Can you work these out from the model? Positions are in its coordinate system, mm. Face numbers are marked on the shaded views. A direction names the side the tool comes from. Coordinates: 2 decimals unless noted, no trailing zeros. Loops run counter-clockwise (first coordinate to the right, second up) from the corner with the lowest first, then second, coordinate; pieces in that order, holes last. Notation, with made-up numbers: (-24, 25) -> (-11, 25) arc R30 cw to (-11, 56) -> close; hole circle Ø1 at (78, 72.5). An arc over 180 degrees is marked (long way). Use one line per item in the form item = value. Start each with the question number.
(1) I'm going to push flat-ended pins straight in: pin 1 (3.5 mm diameter, centred on x = 12, z = 24.5, fed in from -Y); pin 2 (5 mm diameter, centred on x = 9.5, y = 32, fed in from -Z); pin 3 (10 mm diameter, centred on y = -9.5, z = 24, fed in from +X). Where does each tip first touch, or does it pass through?
(2) Imagine slicing it at B-B (z = 8.5). List the corners of the cut face in (x, y) for me, plus the area to 3 significant figures.
(3) On a 3-axis mill with a long thin cutter (end or side, diameter ignored), from which of +Z, -Z, +X, -X, +Y, -Y can I reach the whole of each face in a straight line? I mean the marked faces 1, 2 and 3. Say none if no direction works.
(4) Imagine slicing it at D-D (y = 50.5). List the corners of the cut face in (x, z) for me.
(5) I need wall thicknesses on line 1 (X direction, y = 57.5, z = 17.5); line 2 (X direction, y = 67, z = 16); line 3 (Y direction, x = 6.5, z = 8). Which ranges of each line are inside material? Lowest first, please. Write a range as [from, to].
(6) Imagine slicing it at A-A (z = 16.5). List the corners of the cut face in (x, y) for me.
(7) Imagine slicing it at C-C (x = 6). List the corners of the cut face in (y, z) for me, plus the area to 3 significant figures.
(8) Thinking about a two-plate mould opening in X: for the marked faces 4, 5, 6 and 7, which applies, released by +X, released by -X, zero draft, split by the parting line, or undercut?
```python
from build123d import *

# Parameters (mm, degrees)
BOSS_EXTRU_1_DEPTH                   = 33
ESQUISSE3_R                          = 16.5
BOSS_EXTRU_2_DEPTH                   = 3
ESQUISSE4_R                          = 3
ESQUISSE4_R_2                        = 1.5
ENL_V_MAT_EXTRU_1_DEPTH              = 94.202215967
ESQUISSE5_W                          = 3
ESQUISSE5_H                          = 5
BOSS_EXTRU_3_DEPTH                   = 3
ENL_V_DE_MAT_EXTRU_MINCE2_DEPTH      = 30
ENL_V_DE_MAT_EXTRU_MINCE2_DEPTH_BACK = 90
ESQUISSE2_R                          = 35.75
ESQUISSE2_R_2                        = 15.75


with BuildPart() as part:
    # Esquisse1 → Boss.-Extru.1 (new body)
    with BuildSketch(Plane.XY):
        Polygon((3, 0), (9.5, 9.285714286), (9.5, 68.285714286), (-6.5, 68.285714286), (-6.5, 9.285714286), (0, 0), (0, -20), (3, -20), align=None)
        Polygon((7.5, 9.285714286), (7.5, 65.285714286), (-4.5, 65.285714286), (-4.5, 9.285714286), (1.5, 0.714285714), align=None, mode=Mode.SUBTRACT)
    extrude(amount=BOSS_EXTRU_1_DEPTH)

    # Esquisse3 → Boss.-Extru.2 (add)
    with BuildSketch(Plane(origin=(0, 68.285714286, 0), x_dir=(1, 0, 0), z_dir=(0, 1, 0))):
        with Locations((1.5, -16.5)):
            Circle(ESQUISSE3_R)
    extrude(amount=-BOSS_EXTRU_2_DEPTH)

    # Esquisse4 → Enlèv. mat.-Extru.1 (cut, through all)
    with BuildSketch(Plane.XZ.offset(-65.285714286)):
        with Locations(Location((13.5, 16.5, 0), (0, 0, 270))):
            Circle(ESQUISSE4_R)
        with Locations(Location((12, 8.5, 0), (0, 0, 270))):
            Circle(ESQUISSE4_R_2)
        with Locations(Location((12, 24.5, 0), (0, 0, 90))):
            Circle(ESQUISSE4_R_2)
        Polygon((-12.8, 16.5), (-12.8, 20.5), (-8.8, 20.5), (-8.8, 12.5), (-12.8, 12.5), align=None)
    extrude(amount=-ENL_V_MAT_EXTRU_1_DEPTH, mode=Mode.SUBTRACT)

    # Esquisse5 → Boss.-Extru.3 (add)
    with BuildSketch(Plane.XZ.offset(20)):
        with Locations((1.5, 24.5)):
            Rectangle(ESQUISSE5_W, ESQUISSE5_H)
        with Locations((1.5, 8.5)):
            Rectangle(ESQUISSE5_W, ESQUISSE5_H)
    extrude(amount=BOSS_EXTRU_3_DEPTH)

    # Esquisse2 → Enlèv. de mat.-Extru.-Mince2 (cut, two sides: drawn at the far end of the back side and taken through both)
    with BuildSketch(Plane(origin=(0, 68.285714286, 0), x_dir=(1, 0, 0), z_dir=(0, 1, 0)).offset(-ENL_V_DE_MAT_EXTRU_MINCE2_DEPTH_BACK)):
        with Locations((1.5, -16.5)):
            Circle(ESQUISSE2_R)
        with Locations((1.5, -16.5)):
            Circle(ESQUISSE2_R_2, mode=Mode.SUBTRACT)
    extrude(amount=ENL_V_DE_MAT_EXTRU_MINCE2_DEPTH + ENL_V_DE_MAT_EXTRU_MINCE2_DEPTH_BACK, mode=Mode.SUBTRACT)


solid = part.part
```
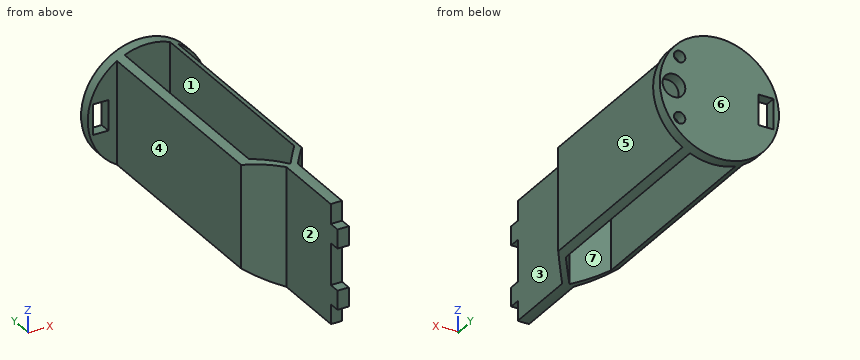
Worked out:
q1.pin_1 = 65.29
q1.pin_2 = 1.94
q1.pin_3 = 3
q2.outline = (-12.07, 65.29) -> (-6.5, 65.29) -> (-6.5, 9.29) -> (0, 0) -> (0, -23) -> (3, -23) -> (3, 0) -> (9.5, 9.29) -> (9.5, 65.29) -> (10.5, 65.29) -> (10.5, 68.29) -> (-12.07, 68.29) -> close; (13.5, 65.29) -> (15.07, 65.29) -> (15.07, 68.29) -> (13.5, 68.29) -> close; hole (-4.5, 9.29) -> (1.5, 0.71) -> (7.5, 9.29) -> (7.5, 65.29) -> (-4.5, 65.29) -> close
q2.area = 402 mm2
q3.face_1 = +Z, -Z
q3.face_2 = +Z, -Z, -X, -Y
q3.face_3 = +Z, -Z, +X, -Y
q4.outline = (-6.5, 2.93) arc R15.75 ccw to (-4.5, 1.94) -> (-4.5, 31.06) arc R15.75 ccw to (-6.5, 30.07) -> close; (7.5, 1.94) arc R15.75 ccw to (9.5, 2.93) -> (9.5, 30.07) arc R15.75 ccw to (7.5, 31.06) -> close
q5.line_1 = [-6.5, -4.5], [7.5, 9.5]
q5.line_2 = [-14.24, -12.8], [-8.8, 10.54], [16.46, 17.24]
q5.line_3 = [5, 7.86], [65.29, 68.29]
q6.outline = (-14.25, 65.29) -> (-12.8, 65.29) -> (-12.8, 68.29) -> (-14.25, 68.29) -> close; (-8.8, 65.29) -> (-6.5, 65.29) -> (-6.5, 9.29) -> (0, 0) -> (0, -20) -> (3, -20) -> (3, 0) -> (9.5, 9.29) -> (9.5, 65.29) -> (10.5, 65.29) -> (10.5, 68.29) -> (-8.8, 68.29) -> close; (16.5, 65.29) -> (17.25, 65.29) -> (17.25, 68.29) -> (16.5, 68.29) -> close; hole (-4.5, 9.29) -> (1.5, 0.71) -> (7.5, 9.29) -> (7.5, 65.29) -> (-4.5, 65.29) -> close
q7.outline = (4.29, 1.41) -> (7.14, 1.41) -> (7.14, 31.59) -> (4.29, 31.59) -> close; (65.29, 1.41) -> (68.29, 1.41) -> (68.29, 31.59) -> (65.29, 31.59) -> close
q7.area = 177 mm2
q8.face_4 = released by -X
q8.face_5 = released by +X
q8.face_6 = zero draft
q8.face_7 = undercut
